Input: part model. Units: mm. Frame: model coordinates. Face numbers are marked on the shaded views. A direction names the side the tool comes from. Coordinates: 2 decimals unless noted, no trailing zeros. Order: outer loops, then holes, each group sorted by start corner. A loop starts at its lowest first (then second) coordinate and runs counter-clockwise, first axis right, second up. Notation, with made-up numbers: (-8.5, -25.75) -> (2.5, -25.75) arc R33 cw to (2.5, 3.25) -> close; hole circle Ø3 at (-8, -29). An arc over 180 degrees is marked (long way). Write each question's results on one line, items separated by ' | '.
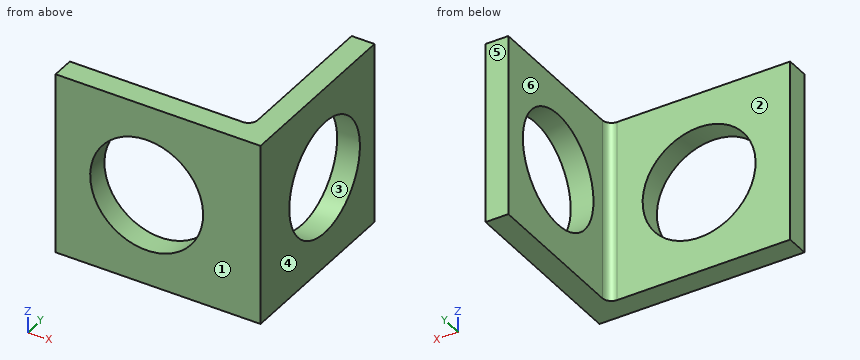
```python
from build123d import *

# Parameters (mm, degrees)
BOSS_EXTRUDE1_DEPTH = 12.7
SKETCH2_R           = 3.937
CUT_EXTRUDE1_DEPTH  = 6.35
SKETCH4_R           = 3.937
CUT_EXTRUDE2_DEPTH  = 6.35
FILLET2_R           = 0.635


with BuildPart() as part:
    # Sketch1 → Boss-Extrude1 (new body)
    with BuildSketch(Plane.XY):
        Polygon((0, 0), (14.2875, 0), (14.2875, 12.7), (12.7, 12.7), (12.7, 1.5875), (0, 1.5875), align=None)
    extrude(amount=BOSS_EXTRUDE1_DEPTH)

    # Sketch2 → Cut-Extrude1 (cut)
    with BuildSketch(Plane.ZY.offset(-12.7)):
        with Locations((6.35, 7.14375)):
            Circle(SKETCH2_R)
    extrude(amount=-CUT_EXTRUDE1_DEPTH, mode=Mode.SUBTRACT)

    # Sketch4 → Cut-Extrude2 (cut)
    with BuildSketch(Plane(origin=(0, 1.5875, 0), x_dir=(1, 0, 0), z_dir=(0, 1, 0))):
        with Locations(Location((6.35, -6.35, 0), (0, 0, 270))):
            Circle(SKETCH4_R)
    extrude(amount=-CUT_EXTRUDE2_DEPTH, mode=Mode.SUBTRACT)

    # Fillet2
    fillet2_edges = [part.edges().sort_by_distance(p)[0] for p in [
        (12.7, 1.5875, 6.35),
    ]]
    fillet(fillet2_edges, radius=FILLET2_R)


solid = part.part
```
(1) Cut plane C-C, the plane y = 3.5. Return loops of the section in (x, z).
Return value:
outline: (12.7, 0) -> (14.29, 0) -> (14.29, 4.86) -> (12.7, 4.86) -> close; (12.7, 7.84) -> (14.29, 7.84) -> (14.29, 12.7) -> (12.7, 12.7) -> close
(2) Cut plane D-D, the plane z = 11.75. Return loops of the section in (x, y) (1 decimal).
Return value:
outline: (0, 0) -> (14.3, 0) -> (14.3, 12.7) -> (12.7, 12.7) -> (12.7, 2.2) arc R0.6 cw to (12.1, 1.6) -> (0, 1.6) -> close
(3) Line query: line 1 along Y through (x, z) = (13.35, 6.35); line 2 along X through (y, z) = (1, 6.35); line 3 along Y through (x, z) = (1, 12). Output: solid intervals per line, ascending. Write a range as from..to.
Return value:
line 1: 0..3.21, 11.08..12.7 | line 2: 0..2.41, 10.29..14.29 | line 3: 0..1.59
(4) Pin query (flat end, axial travel): P1, Ø5, axis at y = 7.5, z = 9, coming from the -X side. Return the tip coordinate at first contact, or that it passes through.
Return value:
P1: x = 12.7
(5) Cut plane B-B, the plane x = 6.35. Return loops of the section in (y, z), plus the area to 3 significant figures.
Return value:
outline: (0, 0) -> (1.59, 0) -> (1.59, 2.41) -> (0, 2.41) -> close; (0, 10.29) -> (1.59, 10.29) -> (1.59, 12.7) -> (0, 12.7) -> close | area: 7.66 mm2
(6) Cut plane A-A, the plane z = 6.35. Return loops of the section in (x, y) (1 decimal).
Return value:
outline: (0, 0) -> (2.4, 0) -> (2.4, 1.6) -> (0, 1.6) -> close; (10.3, 0) -> (14.3, 0) -> (14.3, 3.2) -> (12.7, 3.2) -> (12.7, 2.2) arc R0.6 cw to (12.1, 1.6) -> (10.3, 1.6) -> close; (12.7, 11.1) -> (14.3, 11.1) -> (14.3, 12.7) -> (12.7, 12.7) -> close
(7) Reachability of the marked faces 5 and 6 from +Z, -Z, +X, -X, +Y, -Y: full face, straight path, thin tool, end or side. Return the list, or none.
Return value:
face 5: +Z, -Z, +X, -X, +Y | face 6: +Z, -Z, -X, +Y
(8) Mould query, pull axis Y, two halves, no side actions, for the marked faces 1, 2, 3 and 4. Classes: +Y half, -Y half, draft (parallel to the pull), parting line (faces both ways), or undercut.
Return value:
face 1: -Y half | face 2: +Y half | face 3: undercut | face 4: draft
